from build123d import *

# Parameters (mm, degrees)
BASPROSKE_W        = 3
BASPROSKE_H        = 9
TOOTHCUT_DEPTH     = 14.076696831
TEETHCUTS_COUNT    = 18
TEETHCUTS_ANGLE    = 340
CUT_EXTRUDE1_DEPTH = 14.007462246


with BuildPart() as part:
    # BasProSke → Base-Revolve (revolve)
    with BuildSketch(Plane(origin=(0, 0, 0), x_dir=(1, 0, 0), z_dir=(0, 1, 0)), mode=Mode.PRIVATE) as base_revolve_sk:
        with Locations((1.5, 4.5)):
            Rectangle(BASPROSKE_W, BASPROSKE_H)
    revolve(base_revolve_sk.sketch.rotate(Axis((-10, 0, 0), (1, 0, 0)), 180), axis=Axis((-10, 0, 0), (1, 0, 0)))

    # TooCutSke → ToothCut (cut, through all)
    with BuildSketch(Plane(origin=(0, 0, 0), x_dir=(0, 0, -1), z_dir=(1, 0, 0))):
        with BuildLine():
            ThreePointArc((0.45926649, 6.958861278), (0, 6.974), (-0.45926649, 6.958861278))
            ThreePointArc((-0.45926649, 6.958861278), (-0.743858876, 8.01799277), (-1.365479267, 8.921508366))
            ThreePointArc((-1.365479267, 8.921508366), (0, 9.0254), (1.365479267, 8.921508366))
            ThreePointArc((1.365479267, 8.921508366), (0.743858876, 8.01799277), (0.45926649, 6.958861278))
        make_face()
    toothcut = extrude(amount=TOOTHCUT_DEPTH, mode=Mode.SUBTRACT)

    # TeethCuts: ToothCut ×18 about axis
    teethcuts_axis = Axis((-10, 0, 0), (1, 0, 0))
    for i in range(1, TEETHCUTS_COUNT):
        add(toothcut.rotate(teethcuts_axis, i * TEETHCUTS_ANGLE / (TEETHCUTS_COUNT - 1)), mode=Mode.SUBTRACT)

    # Sketch1 → Cut-Extrude1 (cut, through all)
    with BuildSketch(Plane(origin=(3, 0, 0), x_dir=(0, 0, -1), z_dir=(1, 0, 0))):
        Polygon((0, 3.146558967), (-2.725, 1.573279484), (-2.725, -1.573279484), (0, -3.146558967), (2.725, -1.573279484), (2.725, 1.573279484), align=None)
    extrude(amount=-CUT_EXTRUDE1_DEPTH, mode=Mode.SUBTRACT)


solid = part.part
Verification items for the finished model (mm, model axes). A direction names the side the tool comes from. Round coordinates to 2 decimals unless told otherwise and drop trailing zeros. Order: outer loops, then holes, each group sorted by start corner. A loop starts at its lowest first (then second) coordinate and runs counter-clockwise, first axis right, second up. Notation, with made-up numbers: (67, 2) -> (111, 2) arc R7 cw to (111, 9) -> close; hole circle Ø7 at (53.25, -34). An arc over 180 degrees is marked (long way). Put each result on its own line as item: value.
1) Section check A-A (z = -7.5). Record the cut outline in (x, y), then the cut area to 3 significant figures.
Final values:
outline: (0, -3.38) -> (3, -3.38) -> (3, -1.96) -> (0, -1.96) -> close; (0, -0.75) -> (3, -0.75) -> (3, 0.75) -> (0, 0.75) -> close; (0, 1.96) -> (3, 1.96) -> (3, 3.38) -> (0, 3.38) -> close
area: 13.0 mm^2
2) Mould release check, pull along Y, two halves, no side actions. Record for faces 1 (the cylindrical face through (1.479, 5.651, 5.696)), 2 (the cylindrical face through (1.48, -0.66, 8.03)), 3 (the cylindrical face through (1.479, 3.362, 7.285)), 4 (the cylindrical face through (1.48, -7.28, 3.44)): +Y half, -Y half, draft (parallel to the pull), parting line (faces both ways), or undercut.
Final values:
face 1: +Y half
face 2: undercut
face 3: undercut
face 4: -Y half
3) Material ranges on line 1 (Y direction, x = 1.3, z = -4.25); line 2 (Z direction, x = 2.35, y = 3); line 3 (Z direction, x = 1.15, y = -2.25), recorded low to high.
Final values:
line 1: y = -7.87 to -5.83, -5.53 to 5.53, 5.83 to 7.87
line 2: z = -8.49 to -0.25, 0.25 to 8.49
line 3: z = -7.94 to -1.55, 1.55 to 7.94
4) Section check B-B (y = -7.25). Record the cut outline in (x, z).
Final values:
outline: (0, -4.69) -> (3, -4.69) -> (3, -3.41) -> (0, -3.41) -> close; (0, -2.04) -> (3, -2.04) -> (3, -0.5) -> (0, -0.5) -> close; (0, 0.5) -> (3, 0.5) -> (3, 2.04) -> (0, 2.04) -> close; (0, 3.41) -> (3, 3.41) -> (3, 4.69) -> (0, 4.69) -> close
5) Section check C-C (y = -1). Record the cut outline in (x, z) (3 decimals).
Final values:
outline: (0, -6.902) -> (3, -6.902) -> (3, -2.725) -> (0, -2.725) -> close; (0, 2.725) -> (3, 2.725) -> (3, 6.902) -> (0, 6.902) -> close
6) Depth check by flat-ended pin: pin 1 (4 mm diameter, centred on y = -1, z = -3.5, fed in from -X); pin 2 (1 mm diameter, centred on x = 2, y = 3.5, fed in from +Z); pin 3 (1 mm diameter, centred on x = 2, z = -6, fed in from +Y). Enter the tip coordinate at first touch or a pass-through.
Final values:
pin 1: stops at x = 0
pin 2: stops at z = 8.49
pin 3: stops at y = 5.92
7) Set-up check for faces 5 (the cylindrical face through (1.479, 7.758, -2.046)), 6 (the flat face through (0, -2.1, 2.13)), 7 (the cylindrical face through (1.48, 7.99, 0.73)), 8 (the cylindrical face through (1.479, 2.125, 7.767)): record each of +Z, -Z, +X, -X, +Y, -Y from which the full face is reachable in a straight line by a thin tool's end or side.
Final values:
face 5: +X, -X
face 6: +Z, -Z, -X, +Y, -Y
face 7: +X, -X, +Y
face 8: +Z, +X, -X
8) Section check D-D (z = -2.5). Record the cut outline in (x, y).
Final values:
outline: (0, -6.51) -> (3, -6.51) -> (3, -1.7) -> (0, -1.7) -> close; (0, 1.7) -> (3, 1.7) -> (3, 6.51) -> (0, 6.51) -> close
